```python
from build123d import *

# Parameters (mm, degrees)
SKETCH_W        = 40
SKETCH_H        = 16
SKETCH_R        = 2
PAD_DEPTH       = 1.7
SKETCH001_W     = 7
SKETCH001_H     = 12.5
PAD001_DEPTH    = 6
SKETCH002_W     = 1
SKETCH002_H     = 2
SKETCH002_W_2   = 2
SKETCH002_H_2   = 1
PAD002_DEPTH    = 1
SKETCH004_R     = 1
POCKET_DEPTH    = 6
SKETCH005_W     = 4
SKETCH005_H     = 1.5
POCKET001_DEPTH = 5
SKETCH006_W     = 10.5
SKETCH006_H     = 4
POCKET002_DEPTH = 6
SKETCH007_W     = 3
SKETCH007_H     = 1
POCKET003_DEPTH = 19.501
SKETCH008_W     = 0.5
SKETCH008_H     = 0.5
PAD003_DEPTH    = 5


with BuildPart() as part:
    # Sketch → Pad (new body)
    with BuildSketch(Plane.XY):
        Rectangle(SKETCH_W, SKETCH_H)
        with Locations((-17.5, 5.5)):
            Circle(SKETCH_R, mode=Mode.SUBTRACT)
        with Locations((-17.5, -5.5)):
            Circle(SKETCH_R, mode=Mode.SUBTRACT)
        with Locations((-3, 5.5)):
            Circle(SKETCH_R, mode=Mode.SUBTRACT)
        with Locations((17, 5.5)):
            Circle(SKETCH_R, mode=Mode.SUBTRACT)
    extrude(amount=PAD_DEPTH)

    # Sketch001 (on Face10 of Pad) → Pad001 (new body)
    with BuildSketch(Plane.XY.offset(1.7)):
        Polygon((13.5, 8), (13.5, 2), (12.024086, 2), (11.024086, 1), (9.024086, 1), (8.024086, 2), (5.5, 2), (4.5, 1), (2.5, 1), (1.5, 2), (0.5, 2), (0.5, 8), (1.2, 8), (13.2, 12.105263), (14.2, 13), (16.2, 11.731371), (15.985743, 11.393594), (14.2, 12.526316), (13.5, 11.9), (2.1, 8), (3.5, 8), (4, 8.5), (4.5, 8), align=None)
        with Locations((-12, -0.25)):
            Rectangle(SKETCH001_W, SKETCH001_H)
    extrude(amount=PAD001_DEPTH)

    # Sketch002 (on Face5 of Pad001) → Pad002 (new body)
    with BuildSketch(Plane.XY.offset(1.7)):
        with Locations((-4.24, -1)):
            Rectangle(SKETCH002_W, SKETCH002_H)
        with Locations((-1.7, -1)):
            Rectangle(SKETCH002_W, SKETCH002_H)
        with Locations((18, -1.5)):
            Rectangle(SKETCH002_W_2, SKETCH002_H_2)
        with Locations((18, -4.04)):
            Rectangle(SKETCH002_W_2, SKETCH002_H_2)
    extrude(amount=PAD002_DEPTH)

    # Sketch004 (on Face47 of Pad002) → Pocket (cut)
    with BuildSketch(Plane.XY.offset(7.7)):
        with Locations((3.5, 3)):
            Circle(SKETCH004_R)
        with Locations((10.5, 3)):
            Circle(SKETCH004_R)
    extrude(amount=-POCKET_DEPTH, mode=Mode.SUBTRACT)

    # Sketch005 (on Face61 of Pocket) → Pocket001 (cut)
    with BuildSketch(Plane.XY.offset(7.7)):
        with Locations((-13.5, 2.75)):
            Rectangle(SKETCH005_W, SKETCH005_H)
        with Locations((-13.5, -3.75)):
            Rectangle(SKETCH005_W, SKETCH005_H)
    extrude(amount=-POCKET001_DEPTH, mode=Mode.SUBTRACT)

    # Sketch006 (on Face43 of Pocket001) → Pocket002 (cut)
    with BuildSketch(Plane(origin=(-15.5, 0, 0), x_dir=(0, -1, 0), z_dir=(-1, 0, 0))):
        with Locations((0.25, 4.7)):
            Rectangle(SKETCH006_W, SKETCH006_H)
    extrude(amount=-POCKET002_DEPTH, mode=Mode.SUBTRACT)

    # Sketch007 (on Face44 of Pocket002) → Pocket003 (cut, through all)
    with BuildSketch(Plane.XZ.offset(6.5)):
        with Locations((-14, 6.2)):
            Rectangle(SKETCH007_W, SKETCH007_H)
    extrude(amount=-POCKET003_DEPTH, mode=Mode.SUBTRACT)

    # Sketch008 (on Face77 of Pocket003) → Pad003 (new body)
    with BuildSketch(Plane(origin=(-9.5, 0, 0), x_dir=(0, -1, 0), z_dir=(-1, 0, 0))):
        with Locations((-3.05, 5.45)):
            Rectangle(SKETCH008_W, SKETCH008_H)
        with Locations((-0.85, 5.45)):
            Rectangle(SKETCH008_W, SKETCH008_H)
        with Locations((1.35, 5.45)):
            Rectangle(SKETCH008_W, SKETCH008_H)
        with Locations((3.55, 5.45)):
            Rectangle(SKETCH008_W, SKETCH008_H)
    extrude(amount=PAD003_DEPTH)


solid = part.part
```
Geometry check sheet. Reference: the model listing, model coordinates, mm. A direction names the side the tool comes from. Coordinates: 2 decimals unless noted, no trailing zeros. Order: outer loops, then holes, each group sorted by start corner. A loop starts at its lowest first (then second) coordinate and runs counter-clockwise, first axis right, second up. Notation, with made-up numbers: (50, -23) - (62, -23) arc R29 cw to (62, 13) - close; hole circle Ø1 at (63.5, 29.5). An arc over 180 degrees is marked (long way). Answer as a JSON object with one key per item and string values. Group by question number.
Item 1: Sectioned sample at A-A, the plane x = -10. Record the cut outline in (y, z), and give its area (3 significant figures).
Item 2: Draft check along Y on faces 6 (the face through (7.116, 10.024, 4.658)), 7 (the face through (-9.5, 0, 5)), 8 (the face through (0, 0, 0)), 9 (the face through (4, 8, 1)). Enter one of: +Y half, -Y half, draft (parallel to the pull), parting line (faces both ways), or undercut.
Item 3: Sectioned sample at C-C, the plane x = -3. Record the cut outline in (y, z), and give its area (3 significant figures).
Item 4: Sectioned sample at D-D, the plane x = -17.5. Record the cut outline in (y, z).
Item 5: Sectioned sample at B-B, the plane z = 4.5. Give the number of separate pieces and of enclosed holes in the cut face, and give its area (3 significant figures).
Item 6: Depth check by flat-ended pin: pin 1 Ø3 at (x, z) = (-13.5, 7) entering from +Y; pin 2 Ø0.6 at (x, z) = (10, 3.5) entering from -Y; pin 3 Ø0.5 at (y, z) = (-1.5, 7.5) entering from -X; pin 4 Ø2.5 at (x, y) = (-17.5, -5.5) entering from +Z. Enter the tip coordinate at first touch or a pass-through.
Item 7: Tool access check on faces 1 (the face through (18, -4.54, 2)), 2 (the face through (-12.5, 5.5, 6.2)), 3 (the face through (-15.5, -1, 7)), 4 (the face through (8.531, 1.493, 4.658)), 5 (the face through (-4, 0, 2)). Record the directions out of +Z, -Z, +X, -X, +Y, -Y that give a thin tool (end or side, any length) a straight path to the whole face; none if there is none.
Item 8: Scan lines: probe 1 along Z at (x, y) = (-10, -3.25); probe 2 along Y at (x, z) = (17, 1); probe 3 along Y at (x, z) = (10.5, 3.2). Record each from-to range of solid material in increasing order.
Resolved:
{
 "1": {"outline": "(-8, 0) - (8, 0) - (8, 1.7) - (6, 1.7) - (6, 7.7) - (-6.5, 7.7) - (-6.5, 1.7) - (-8, 1.7) - close; (-3.8, 5.2) - (-3.3, 5.2) - (-3.3, 5.7) - (-3.8, 5.7) - close; (-1.6, 5.2) - (-1.1, 5.2) - (-1.1, 5.7) - (-1.6, 5.7) - close; (0.6, 5.2) - (1.1, 5.2) - (1.1, 5.7) - (0.6, 5.7) - close; (2.8, 5.2) - (3.3, 5.2) - (3.3, 5.7) - (2.8, 5.7) - close; hole (-5.5, 2.7) - (5, 2.7) - (5, 6.7) - (-5.5, 6.7) - close", "area": "61.2 mm^2"},
 "2": {"face 6": "+Y half", "face 7": "undercut", "face 8": "draft", "face 9": "undercut"},
 "3": {"outline": "(-8, 0) - (3.5, 0) - (3.5, 1.7) - (-8, 1.7) - close; (7.5, 0) - (8, 0) - (8, 1.7) - (7.5, 1.7) - close", "area": "20.4 mm^2"},
 "4": {"outline": "(-8, 0) - (-7.5, 0) - (-7.5, 1.7) - (-8, 1.7) - close; (-3.5, 0) - (3.5, 0) - (3.5, 1.7) - (-3.5, 1.7) - close; (7.5, 0) - (8, 0) - (8, 1.7) - (7.5, 1.7) - close"},
 "5": {"separate pieces": "2", "enclosed holes": "2", "area": "107 mm^2"},
 "6": {"pin 1": "y = 6", "pin 2": "y = 1", "pin 3": "x = -15.5", "pin 4": "through"},
 "7": {"face 1": "+Z, +X, -Y", "face 2": "-X, +Y, -Y", "face 3": "+Z, -X, +Y, -Y", "face 4": "+Z, -Y", "face 5": "+Z, +X, +Y"},
 "8": {"probe 1": "0 to 2.7, 6.7 to 7.7", "probe 2": "-8 to 3.5, 7.5 to 8", "probe 3": "1 to 2, 4 to 8, 10.87 to 11.18"}
}
